from build123d import *

# Parameters (mm, degrees)
F0_W     = 15.24
F0_H     = 243.84
F1_DEPTH = 0.254
F2_W     = 15.24
F2_H     = 0.254
F3_DEPTH = 243.332
F4_W     = 15.249304
F4_H     = 243.84
F5_DEPTH = 0.254
F6_W     = 2.54
F6_H     = 243.332
F7_DEPTH = 243.332


with BuildPart() as f1:
    # F0 (on Front) → F1 (new body)
    with BuildSketch(Plane.XZ):
        with Locations((7.62, -121.92)):
            Rectangle(F0_W, F0_H)
    extrude(amount=F1_DEPTH)

    # F2 (on face) → F3 (join)
    with BuildSketch(Plane.XZ.offset(0.254)):
        with Locations((7.62, -0.127)):
            Rectangle(F2_W, F2_H)
        with Locations((7.62, -243.713)):
            Rectangle(F2_W, F2_H)
    extrude(amount=F3_DEPTH)

    # F4 (on face) → F5 (join)
    with BuildSketch(Plane.XZ.offset(243.586)):
        with Locations((7.624652, -121.92)):
            Rectangle(F4_W, F4_H)
    extrude(amount=F5_DEPTH)

    # F6 (on face) → F7 (join)
    with BuildSketch(Plane.XY.offset(-243.586)):
        with Locations((13.97, -121.92)):
            Rectangle(F6_W, F6_H)
        with Locations((7.62, -121.92)):
            Rectangle(F6_W, F6_H)
        with Locations((1.27, -121.92)):
            Rectangle(F6_W, F6_H)
    extrude(amount=F7_DEPTH)


solid = f1.part
Read the model definition and answer for the solid it produces. Units are mm, in the model's axes. A direction names the side the tool comes from. Round coordinates to 2 decimals unless told otherwise and drop trailing zeros. Loops run counter-clockwise (first coordinate to the right, second up) from the corner with the lowest first, then second, coordinate; pieces in that order, holes last. Notation, with made-up numbers: (57, 52) - (77, 52) arc R26 cw to (77, 73) - close; hole circle Ø2 at (86, 19). An arc over 180 degrees is marked (long way). One line per question, with ' | ' between items. Start each with the question number.
Q1. For faces 1 (the flat face through (2.54, -124, -124)), 2 (the flat face through (8, -243.84, -120)), determine the directions among +Z, -Z, +X, -X, +Y, -Y from which every point of the face is accessible in a straight line to the end or side of a thin tool.
Q2. Section B-B on y = -164.5 is taken. Give the vertices of the cut face in (x, z), plus the area to 3 significant figures.
Q3. For a pull along Z with two mould halves and no side action, classify faces 3 (the flat face through (15.24, -123, -124)), 4 (the flat face through (8, -120, -243.84)), 5 (the flat face through (8.89, -124, -124)) as +Z half, -Z half, draft (parallel to the pull), parting line (faces both ways), or undercut.
Q4. A flat-ended cylindrical pin translates along its axis: pin 1 (12 mm diameter, centred on y = -69, z = -153, fed in from +X). Find the tip coordinate at first contact, or state that the pin passes through.
Q5. Section A-A on z = -82 is taken. Count the separate pieces of the cut face and the enclosed holes in it, plus the area to 3 significant figures.
Q6. Find the intervals of material crossed by L1, parallel to X at y = -152, z = -162; L2, parallel to Y at x = 5.5, z = -101, in increasing order.
Established:
1) face 1: none | face 2: +Z, -Z, +X, -X, -Y
2) outline: (0, -243.84) - (15.24, -243.84) - (15.24, 0) - (0, 0) - close; hole (2.54, -243.59) - (6.35, -243.59) - (6.35, -0.25) - (2.54, -0.25) - close; hole (8.89, -243.59) - (12.7, -243.59) - (12.7, -0.25) - (8.89, -0.25) - close | area: 1,860 mm²
3) face 3: draft | face 4: -Z half | face 5: undercut
4) pin 1: x = 15.24
5) separate pieces: 1 | enclosed holes: 2 | area: 1,860 mm²
6) L1: 0 to 2.54, 6.35 to 8.89, 12.7 to 15.24 | L2: -243.84 to -243.59, -0.25 to 0
